Input: part model. Units: mm. Frame: model coordinates. Face numbers are marked on the shaded views. A direction names the side the tool comes from. Coordinates: 2 decimals unless noted, no trailing zeros. Write each loop counter-clockwise with the first axis right and the second up, starting at its lowest first coordinate (ties: lowest second). Pieces come first, ordered by that corner, then holes. Notation, with made-up numbers: (35, 43.25) - (42, 43.25) arc R11 cw to (42, 51.25) - close; hole circle Ø9 at (53.5, -27). An arc over 180 degrees is marked (long way). Put each result on its own line as item: value. Start each with the question number.
1. Cut plane D-D, the plane z = -7. Count the separate pieces of the cut face and the enclosed holes in it, and give its area (3 significant figures).
2. Access query for the marked faces 1, 2 and 3. Directions: +Z, -Z, +X, -X, +Y, -Y. A direction counts if a zero-diameter tool reaches every point of the face in a straight line with its end or side. Return the directions, or none.
3. Cut plane A-A, the plane x = -17.5. Return loops of the section in (y, z).
4. Cut plane C-C, the plane y = -5.5. Return loops of the section in (x, z).
5. Pin query (flat end, axial travel): pin 1 (2.5 mm diameter, centred on x = -18, y = -28, fed in from +Z); pin 2 (2 mm diameter, centred on x = 4, y = -11.5, fed in from -Z); pin 3 (10 mm diameter, centred on y = -18.5, z = -9.5, fed in from -X). Return the tip coordinate at first contact, or that it passes through.
6. Cut plane B-B, the plane y = -22.5. Return loops of the section in (x, z).
7. Pull-direction query (Z, two-part tool) for the marked faces 4, 5 and 6; classes: released by +Z, released by -Z, zero draft, split by the parting line, or undercut.
8. Line query: line 1 (X direction, y = -7.5, z = 0); line 2 (Y direction, x = -11.5, z = 2.5); line 3 (Y direction, x = -20, z = -8.5). Output: solid intervals per line, ascending.
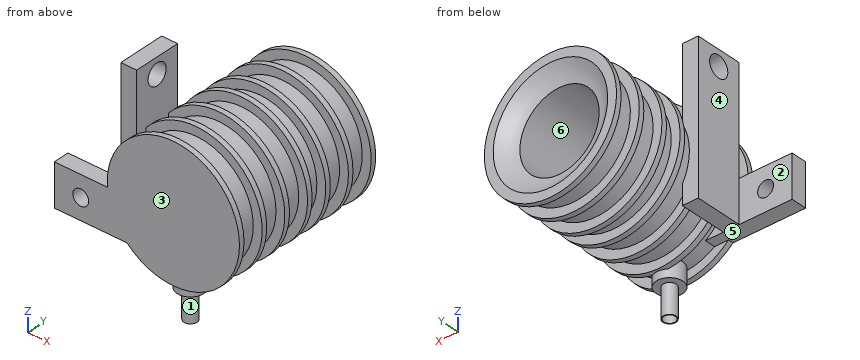
from build123d import *

# Parameters (mm, degrees)
CROQUIS2_R              = 7.5
CORTAR_EXTRUIR1_DEPTH   = 24
SALIENTE_EXTRUIR1_DEPTH = 3
SALIENTE_EXTRUIR2_DEPTH = 3
CROQUIS7_R              = 1.5
CORTAR_EXTRUIR3_DEPTH   = 13
CROQUIS8_R              = 1.5
CORTAR_EXTRUIR4_DEPTH   = 13
CROQUIS9_R              = 2.5
SALIENTE_EXTRUIR3_DEPTH = 13
CROQUIS10_R             = 1.104312036
CORTAR_EXTRUIR5_DEPTH   = 13
CROQUIS13_R             = 2.5
CROQUIS13_R_2           = 1.25
CORTAR_EXTRUIR6_DEPTH   = 5.5
CROQUIS15_W             = 10
CROQUIS15_H             = 8
SALIENTE_EXTRUIR4_DEPTH = 3
CROQUIS16_R             = 1.5
CORTAR_EXTRUIR7_DEPTH   = 30
CROQUIS17_R             = 1.5
SALIENTE_EXTRUIR5_DEPTH = 3
CROQUIS18_W             = 2
CROQUIS18_H             = 9
CORTAR_EXTRUIR11_DEPTH  = 3
CROQUIS19_R             = 2
CORTAR_EXTRUIR12_DEPTH  = 33


with BuildPart() as part:
    # Croquis1 → Revolución1 (revolve)
    with BuildSketch(Plane.XY, mode=Mode.PRIVATE) as revoluci_n1_sk:
        with BuildLine():
            Line((-10.818667505, 0), (-12.5, 0))
            Line((-12.5, 0), (-12.5, -1))
            Line((-12.5, -1), (-10.818667505, -1))
            Line((-10.818667505, -1), (-10.818667505, -5))
            Line((-10.818667505, -5), (-12.5, -5))
            Line((-12.5, -5), (-12.5, -6))
            Line((-12.5, -6), (-10.818667505, -6))
            Line((-10.818667505, -6), (-10.818667505, -10))
            Line((-10.818667505, -10), (-12.5, -10))
            Line((-12.5, -10), (-12.5, -11))
            Line((-12.5, -11), (-10.818667505, -11))
            Line((-10.818667505, -11), (-10.818667505, -14))
            Line((-10.818667505, -14), (-12.5, -14))
            Line((-12.5, -14), (-12.5, -15))
            Line((-12.5, -15), (-10.818667505, -15))
            Line((-10.818667505, -15), (-10.818667505, -19))
            Line((-10.818667505, -19), (-12.5, -19))
            Line((-12.5, -19), (-12.5, -20))
            Line((-12.5, -20), (-10.818667505, -20))
            Line((-10.818667505, -20), (-10.818667505, -24))
            Line((-10.818667505, -24), (-12.5, -24))
            Line((-12.5, -24), (-12.5, -25))
            Line((-12.5, -25), (-10.818667505, -25))
            Line((-10.818667505, -25), (-10.818667505, -29))
            Line((-10.818667505, -29), (-12.5, -29))
            Line((-12.5, -29), (-12.5, -30))
            Line((-12.5, -30), (0, -30))
            Line((0, -30), (0, -2))
            Line((0, -2), (-7.5, -2))
            add(Edge.make_bspline(
                [(-10.818667505, 0), (-9.258756579, -1.530453888), (-7.5, -2)],
                knots=[0, 0, 0, 0.398472736, 0.398472736, 0.398472736], degree=2))
        make_face()
    revolve(revoluci_n1_sk.sketch.rotate(Axis((0, -2, 0), (0, -1, 0)), 270), axis=Axis((0, -2, 0), (0, -1, 0)))

    # Croquis2 → Cortar-Extruir1 (cut)
    with BuildSketch(Plane(origin=(0, 0, 0), x_dir=(1, 0, 0), z_dir=(0, 1, 0))):
        with Locations(Location((0, 0, 0), (0, 0, 270))):
            Circle(CROQUIS2_R)
    extrude(amount=-CORTAR_EXTRUIR1_DEPTH, mode=Mode.SUBTRACT)

    # Croquis4 → Saliente-Extruir1 (add)
    with BuildSketch(Plane.ZY.offset(12.5)):
        Polygon((-8.915161304, -27), (10.818667505, -27), (21.084838696, -27), (21.084838696, -18), (-8.915161304, -18), align=None)
    extrude(amount=-SALIENTE_EXTRUIR1_DEPTH)

    # Croquis6 → Saliente-Extruir2 (add)
    with BuildSketch(Plane.XZ.offset(30)):
        Polygon((-12.5, -8.915161304), (-21.5, -8.915161304), (-21.5, -0.915161304), (-12.5, -0.915161304), (-4.999981801, -0.915161304), (-4.999981801, -8.915161304), align=None)
    extrude(amount=-SALIENTE_EXTRUIR2_DEPTH)

    # Croquis7 → Cortar-Extruir3 (cut)
    with BuildSketch(Plane.XZ.offset(30)):
        with Locations(Location((-18, -4.915161304, 0), (0, 0, 270))):
            Circle(CROQUIS7_R)
    extrude(amount=-CORTAR_EXTRUIR3_DEPTH, mode=Mode.SUBTRACT)

    # Croquis8 → Cortar-Extruir4 (cut)
    with BuildSketch(Plane.ZY.offset(12.5)):
        with Locations((17.584838696, -22.5)):
            Circle(CROQUIS8_R)
    extrude(amount=-CORTAR_EXTRUIR4_DEPTH, mode=Mode.SUBTRACT)

    # Croquis9 → Saliente-Extruir3 (add)
    with BuildSketch(Plane.XY.offset(-19.5)):
        with Locations(Location((0.659333752, -27, 0), (0, 0, 126.869897752))):
            Circle(CROQUIS9_R)
    extrude(amount=SALIENTE_EXTRUIR3_DEPTH)

    # Croquis10 → Cortar-Extruir5 (cut)
    with BuildSketch(Plane(origin=(0, 0, -19.5), x_dir=(-1, 0, 0), z_dir=(0, 0, -1))):
        with Locations((-0.659333752, -27)):
            Circle(CROQUIS10_R)
    extrude(amount=-CORTAR_EXTRUIR5_DEPTH, mode=Mode.SUBTRACT)

    # Croquis13 → Cortar-Extruir6 (cut)
    with BuildSketch(Plane(origin=(0, 0, -19.5), x_dir=(-1, 0, 0), z_dir=(0, 0, -1))):
        with Locations((-0.659333752, -27)):
            Circle(CROQUIS13_R)
        with Locations((-0.659333752, -27)):
            Circle(CROQUIS13_R_2, mode=Mode.SUBTRACT)
    extrude(amount=-CORTAR_EXTRUIR6_DEPTH, mode=Mode.SUBTRACT)

    # Croquis15 → Saliente-Extruir4 (add)
    with BuildSketch(Plane(origin=(0, -27, 0), x_dir=(1, 0, 0), z_dir=(0, 1, 0))):
        with Locations((-17.5, 4.915161304)):
            Rectangle(CROQUIS15_W, CROQUIS15_H)
    extrude(amount=-SALIENTE_EXTRUIR4_DEPTH)

    # Croquis16 → Cortar-Extruir7 (cut)
    with BuildSketch(Plane(origin=(0, -27, 0), x_dir=(1, 0, 0), z_dir=(0, 1, 0))):
        with Locations(Location((-17.5, 4.915161304, 0), (0, 0, 270))):
            Circle(CROQUIS16_R)
    extrude(amount=-CORTAR_EXTRUIR7_DEPTH, mode=Mode.SUBTRACT)

    # Croquis17 → Saliente-Extruir5 (add)
    with BuildSketch(Plane.ZY.offset(12.5)):
        Polygon((19.084838696, -18), (-8.915161304, -18), (-8.915161304, -27), (-0.915161304, -27), (19.084838696, -27), (19.084838696, -22.5), align=None)
        with Locations((17.584838696, -22.5)):
            Circle(CROQUIS17_R, mode=Mode.SUBTRACT)
        with Locations((17.584838696, -22.5)):
            Circle(CROQUIS17_R)
    extrude(amount=-SALIENTE_EXTRUIR5_DEPTH)

    # Croquis18 → Cortar-Extruir11 (cut)
    with BuildSketch(Plane.ZY.offset(12.5)):
        with Locations((20.084838696, -22.5)):
            Rectangle(CROQUIS18_W, CROQUIS18_H)
    extrude(amount=-CORTAR_EXTRUIR11_DEPTH, mode=Mode.SUBTRACT)

    # Croquis19 → Cortar-Extruir12 (cut)
    with BuildSketch(Plane.ZY.offset(12.5)):
        with Locations((16.084838696, -22.5)):
            Circle(CROQUIS19_R)
    extrude(amount=-CORTAR_EXTRUIR12_DEPTH, mode=Mode.SUBTRACT)


solid = part.part
Report:
1. separate pieces: 1
1. enclosed holes: 3
1. area: 443 mm^2
2. face 1: -Z
2. face 2: +Z, -Z, -X, +Y
2. face 3: +Z, -Z, +X, -X, -Y
3. outline: (-30, -8.92) - (-27, -8.92) - (-27, -6.42) - (-30, -6.42) - close; (-30, -3.42) - (-27, -3.42) - (-27, -0.92) - (-30, -0.92) - close
4. outline: circle Ø25 at (0, 0); hole circle Ø15 at (0, 0)
5. pin 1: stops at z = -0.92
5. pin 2: stops at z = -12.1
5. pin 3: stops at x = -12.5
6. outline: (-12.5, -8.92) - (-9.5, -8.92) - (-9.5, -5.18) arc R10.82 ccw (long way) to (-9.5, 5.18) - (-9.5, 14.08) - (-12.5, 14.08) - close; (-12.5, 18.08) - (-9.5, 18.08) - (-9.5, 19.08) - (-12.5, 19.08) - close; hole circle Ø15 at (0, 0)
7. face 4: zero draft
7. face 5: released by -Z
7. face 6: undercut
8. line 1: x = -10.82 to -7.5, 7.5 to 10.82
8. line 2: y = -30 to -29, -27 to -18, -15 to -14, -11 to -10, -6 to -5, -1 to 0
8. line 3: y = -30 to -27
